Part print with two shaded views. Sizes in mm from the minimum x, y, z corner. Round coordinates to 2 decimals unless told otherwise and drop trailing zeros. Write each loop counter-clockwise with the first axis right and the second up, starting at its lowest first coordinate (ties: lowest second). Pieces come first, ordered by that corner, then holes. Notation, with made-up numbers: M 35.25,-37.5 L 48.25,-37.5 A23 cw 48.25,-7.5 Z; hole C 34.25,-30 d4. An arc over 180 degrees is marked long. One line per question, with ' | ' between items. Start each with the question number.
1) Saw through at B-B (x = 60). List the corners of the cut face in (y, z), plus the area to 3 significant figures.
2) Saw through at A-A (y = 20). List the corners of the cut face in (x, z).
3) Wall check: probe 1 along X at (y, z) = (23.5, 2.3); probe 2 along Y at (x, z) = (290, 3.15); probe 3 along X at (y, z) = (14.5, 1.6). Give the ranges that are in metal, low to high. Write a range as [from, to].
4) Saw through at C-C (z = 0.8). List the corners of the cut face in (x, y), plus the area to 3 significant figures.
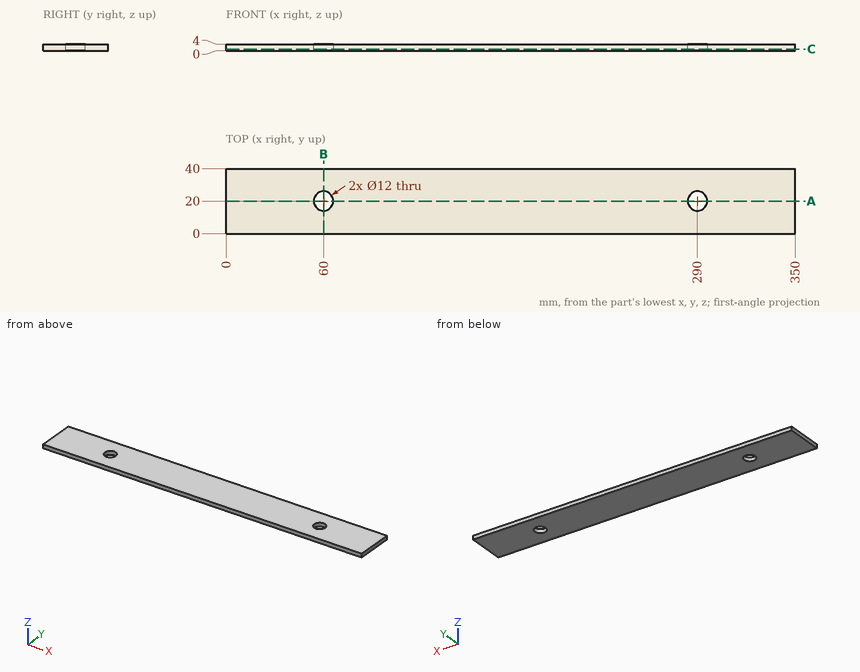
Answer key:
1) outline: M 0,0 L 14,0 L 14,4 L 0,4 Z; M 26,0 L 40,0 L 40,4 L 26,4 Z | area: 112 mm2
2) outline: M 0,0 L 54,0 L 54,4 L 0,4 Z; M 66,0 L 284,0 L 284,4 L 66,4 Z; M 296,0 L 350,0 L 350,4 L 296,4 Z
3) probe 1: x = [0, 55.13], [64.87, 285.13], [294.87, 350] | probe 2: y = [0, 14], [26, 40] | probe 3: x = [0, 57.6], [62.4, 287.6], [292.4, 350]
4) outline: M 0,0 L 350,0 L 350,40 L 0,40 Z; hole C 60,20 d12; hole C 290,20 d12 | area: 13,800 mm2
